Build history of the part. All positions in model axes, mm. A direction names the side the tool comes from. Give positions to 0.01 mm unless a question says otherwise; leave off trailing zeros. Order: outer loops, then holes, each group sorted by start corner. A loop starts at its lowest first (then second) coordinate and runs counter-clockwise, first axis right, second up. Notation, with made-up numbers: (76, 81.25) - (94, 81.25) arc R24 ccw to (94, 96.25) - close; hole circle Ø6 at (77, 21.5). An arc over 180 degrees is marked (long way). One line per item, written item: value.
```python
from build123d import *

# Parameters (mm, degrees)
SKETCH1_R               = 12.35
BOSS_EXTRUDE1_DEPTH     = 20
SKETCH1_5_R             = 12.35
SKETCH1_5_R_2           = 4.5
SKETCH1_5_R_3           = 1.35
BOSS_EXTRUDE2_DEPTH     = 1.7
CUT_EXTRUDE1_DEPTH      = 32
CUT_EXTRUDE1_DEPTH_BACK = 30
SKETCH2_R               = 1.9


with BuildPart() as part:
    # Sketch1 → Boss-Extrude1 (new body)
    with BuildSketch(Plane(origin=(0, 0, 0), x_dir=(1, 0, 0), z_dir=(0, 1, 0))):
        with BuildLine():
            Line((-25, -14.85), (0, -14.85))
            ThreePointArc((0, -14.85), (10.500535701, 10.500535701), (-14.85, 0))
            Line((-14.85, 0), (-25, -2.85))
            Line((-25, -2.85), (-25, -14.85))
        make_face()
        with Locations(Location((0, 0, 0), (0, 0, 270))):
            Circle(SKETCH1_R, mode=Mode.SUBTRACT)
    boss_extrude1 = extrude(amount=BOSS_EXTRUDE1_DEPTH)

    # Sketch1_5 → Boss-Extrude2 (add)
    with BuildSketch(Plane(origin=(0, 0, 0), x_dir=(1, 0, 0), z_dir=(0, 1, 0))):
        with Locations(Location((0, 0, 0), (0, 0, 270))):
            Circle(SKETCH1_5_R)
        with Locations(Location((0, 0, 0), (0, 0, 270))):
            Circle(SKETCH1_5_R_2, mode=Mode.SUBTRACT)
        with Locations(Location((0, -8.35, 0), (0, 0, 270))):
            Circle(SKETCH1_5_R_3, mode=Mode.SUBTRACT)
        with Locations(Location((0, 8.35, 0), (0, 0, 270))):
            Circle(SKETCH1_5_R_3, mode=Mode.SUBTRACT)
    extrude(amount=BOSS_EXTRUDE2_DEPTH)

    # Mirror1: Boss-Extrude1 across plane
    add(boss_extrude1.mirror(Plane(origin=(0, 0, 0), x_dir=(0, 0, 1), z_dir=(1, 0, 0))))

    # Sketch2 → Cut-Extrude1 (cut, two sides: drawn at the far end of the back side and taken through both)
    with BuildSketch(Plane(origin=(0, 0, 0), x_dir=(0, 0, -1), z_dir=(1, 0, 0)).offset(-CUT_EXTRUDE1_DEPTH_BACK)):
        with Locations(Location((-8.85, 4, 0), (0, 0, 180))):
            Circle(SKETCH2_R)
        with Locations(Location((-8.85, 16, 0), (0, 0, 180))):
            Circle(SKETCH2_R)
    extrude(amount=CUT_EXTRUDE1_DEPTH + CUT_EXTRUDE1_DEPTH_BACK, mode=Mode.SUBTRACT)


solid = part.part
```
(1) Drill centre lines: line 1 (Y direction, x = -10, z = 8.85); line 2 (Z direction, x = 0.5, y = 12); line 3 (Y direction, x = 22, z = 10.25). Where is each one in solid material? Low to high.
Completed:
line 1: 0 to 2.1, 5.9 to 14.1, 17.9 to 20
line 2: -14.84 to -12.34, 12.34 to 14.85
line 3: 0 to 2.72, 5.28 to 14.72, 17.28 to 20
(2) Pin check, flat tips, straight feed: P1, Ø4, axis at y = 10.5, z = -11, coming from the +X side; P2, Ø10, axis at x = -3.5, z = -8, coming from the -Y side; P3, Ø3, axis at y = 4, z = 8.85, coming from the +X side; P4, Ø8, axis at x = -8, y = 11, coming from the -Z side. Stop position of each tip, or through.
Completed:
P1: x = 11.81
P2: y = 0
P3: through
P4: z = -14.3
(3) Slice it at A-A, the plane x = 0. Give the cut face in (y, z).
Completed:
outline: (0, -14.85) - (20, -14.85) - (20, -12.35) - (1.7, -12.35) - (1.7, -9.7) - (0, -9.7) - close; (0, -7) - (1.7, -7) - (1.7, -4.5) - (0, -4.5) - close; (0, 4.5) - (1.7, 4.5) - (1.7, 7) - (0, 7) - close; (0, 9.7) - (1.7, 9.7) - (1.7, 12.35) - (20, 12.35) - (20, 14.85) - (0, 14.85) - close
(4) 3-axis set-ups, long thin cutter, end or side, ignore diameter. For faces 4 (the face through (3.71, 10.72, 11.78)), 5 (the face through (-25, 10, 9)): which of +Z, -Z, +X, -X, +Y, -Y reach the whole face in a straight line?
Completed:
face 4: +Y
face 5: +Z, -Z, -X, +Y, -Y
(5) Slice it at C-C, the plane y = 5. Give the cut face in (x, z), and give its area (3 significant figures).
Completed:
outline: (-25, 2.85) - (-14.85, 0) arc R14.85 ccw to (14.85, 0) - (25, 2.85) - (25, 7.23) - (10.01, 7.23) arc R12.35 cw (long way) to (-10.01, 7.23) - (-25, 7.23) - close; (-25, 10.47) - (-6.56, 10.47) arc R12.35 cw to (6.56, 10.47) - (25, 10.47) - (25, 14.85) - (-25, 14.85) - close
area: 474 mm²
(6) Pull direction Y, two halves, no side cores. Call faces 1 (the face through (17.51, 16.728, 10.605)), 2 (the face through (0, 20, 13)), 3 (the face through (0.06, 0.84, -9.7)): +Y half, -Y half, draft (parallel to the pull), parting line (faces both ways), or undercut.
Completed:
face 1: undercut
face 2: +Y half
face 3: draft
(7) Slice it at B-B, the plane z = 8.85. Give the cut face in (x, y).
Completed:
outline: (-25, 0) - (-1.25, 0) - (-1.25, 1.7) - (-8.61, 1.7) - (-8.61, 2.1) - (-25, 2.1) - close; (-25, 5.9) - (-8.61, 5.9) - (-8.61, 14.1) - (-25, 14.1) - close; (-25, 17.9) - (-8.61, 17.9) - (-8.61, 20) - (-25, 20) - close; (1.25, 0) - (25, 0) - (25, 2.1) - (8.61, 2.1) - (8.61, 1.7) - (1.25, 1.7) - close; (8.61, 5.9) - (25, 5.9) - (25, 14.1) - (8.61, 14.1) - close; (8.61, 17.9) - (25, 17.9) - (25, 20) - (8.61, 20) - close
(8) Slice it at D-D, the plane z = -3.25. Give the cut face in (x, y).
Completed:
outline: (-14.49, 0) - (-3.11, 0) - (-3.11, 1.7) - (-11.91, 1.7) - (-11.91, 20) - (-14.49, 20) - close; (3.11, 0) - (14.49, 0) - (14.49, 20) - (11.91, 20) - (11.91, 1.7) - (3.11, 1.7) - close
